Build history of the part. All positions in model axes, mm. A direction names the side the tool comes from. Give positions to 0.01 mm unless a question says otherwise; leave off trailing zeros. Order: outer loops, then holes, each group sorted by start corner. A loop starts at its lowest first (then second) coordinate and runs counter-clockwise, first axis right, second up. Notation, with made-up numbers: (51.5, -0.75) -> (95.5, -0.75) arc R10 ccw to (95.5, 16.25) -> close; hole circle Ø1 at (-30.75, -28). An arc over 180 degrees is marked (long way). One line per item, written item: value. Start each with the question number.
(1) Which spindle directions (+Z, -Z, +X, -X, +Y, -Y) get a long thin tool onto all of the face, cutting with end or side? Do faces 1 (the flat face through (272.5, 276, 290)), 2 (the flat face through (272.5, 324, 290)), 3 (the cylindrical face through (269.78, 284.43, 289.96)), 4 (the flat face through (267, 326, 307)), 5 (the flat face through (269.5, 300, 310)). Say none if no direction does.
(2) Two-plate mould, pull along Z, no slides. Class faces 6 (the flat face through (272.5, 300, 290)), 7 (the flat face through (268, 300, 287)), 8 (the flat face through (270, 300, 293)): +Z half, -Z half, draft (parallel to the pull), parting line (faces both ways), or undercut.
(3) Probe line 1 (Y direction, x = 267.25, z = 300); line 2 (Z direction, x = 265.85, y = 300); line 3 (Y direction, x = 265.2, z = 293.25). List the from-to ranges inside material, lowest first.
(4) Saw through at C-C on y = 300. Give the cut face in (x, z).
(5) Saw through at A-A on y = 283. Give the cut face in (x, z).
(6) Pin check, flat tips, straight feed: pin 1 (4 mm diameter, centred on y = 311.69, z = 293.25, fed in from +X); pin 2 (3 mm diameter, centred on y = 303.5, z = 309, fed in from +X); pin 3 (3.5 mm diameter, centred on y = 276, z = 289, fed in from +X); pin 4 (2 mm diameter, centred on x = 270.7, y = 317, fed in from +Z). Stop position of each tip, or through.
(7) Saw through at B-B on z = 313.5. Give the cut face in (x, y).
(8) Saw through at D-D on x = 267.5. Give the cut face in (y, z).
```python
from build123d import *

# Parameters (mm, degrees)
SKETCH1_W           = 39.5
SKETCH1_H           = 52
SKETCH1_R           = 1.45
BOSS_EXTRUDE1_DEPTH = 5.5
SKETCH2_R           = 7.6
CUT_EXTRUDE1_DEPTH  = 5.5
SKETCH3_W           = 8.5
SKETCH3_H           = 52
BOSS_EXTRUDE2_DEPTH = 6
SKETCH4_R           = 5.05
SKETCH4_R_2         = 1.7
BOSS_EXTRUDE3_DEPTH = 6
SKETCH5_R           = 5.05
SKETCH5_R_2         = 1.7
BOSS_EXTRUDE4_DEPTH = 6
SKETCH6_R           = 1.7
CUT_EXTRUDE2_DEPTH  = 6


with BuildPart() as part:
    # Sketch1 → Boss-Extrude1 (new body)
    with BuildSketch(Plane(origin=(264, 0, 0), x_dir=(0, 0, -1), z_dir=(1, 0, 0))):
        with Locations((-306.75, 300)):
            Rectangle(SKETCH1_W, SKETCH1_H)
        with Locations((-313.5, 300)):
            Circle(SKETCH1_R, mode=Mode.SUBTRACT)
        with Locations((-293.25, 311.691342951)):
            Circle(SKETCH1_R, mode=Mode.SUBTRACT)
        with Locations((-293.25, 288.308657049)):
            Circle(SKETCH1_R, mode=Mode.SUBTRACT)
    extrude(amount=BOSS_EXTRUDE1_DEPTH)

    # Sketch2 → Cut-Extrude1 (cut)
    with BuildSketch(Plane(origin=(264, 0, 0), x_dir=(0, 0, -1), z_dir=(1, 0, 0))):
        with Locations((-300, 300)):
            Circle(SKETCH2_R)
    extrude(amount=CUT_EXTRUDE1_DEPTH, mode=Mode.SUBTRACT)

    # Sketch3 → Boss-Extrude2 (add)
    with BuildSketch(Plane.XY.offset(287)):
        with Locations((268.25, 300)):
            Rectangle(SKETCH3_W, SKETCH3_H)
    extrude(amount=BOSS_EXTRUDE2_DEPTH)

    # Sketch4 → Boss-Extrude3 (add)
    with BuildSketch(Plane.XY.offset(287)):
        with Locations((270.7, 283)):
            Circle(SKETCH4_R)
        with Locations((270.7, 283)):
            Circle(SKETCH4_R_2, mode=Mode.SUBTRACT)
    extrude(amount=BOSS_EXTRUDE3_DEPTH)

    # Sketch5 → Boss-Extrude4 (add)
    with BuildSketch(Plane.XY.offset(287)):
        with Locations((270.7, 317)):
            Circle(SKETCH5_R)
        with Locations((270.7, 317)):
            Circle(SKETCH5_R_2, mode=Mode.SUBTRACT)
    extrude(amount=BOSS_EXTRUDE4_DEPTH)

    # Sketch6 → Cut-Extrude2 (cut)
    with BuildSketch(Plane.XY.offset(287)):
        with Locations(Location((270.7, 283, 0), (0, 0, 225.099127844))):
            Circle(SKETCH6_R)
        with Locations(Location((270.7, 317, 0), (0, 0, 225.099127844))):
            Circle(SKETCH6_R)
    extrude(amount=CUT_EXTRUDE2_DEPTH, mode=Mode.SUBTRACT)


solid = part.part
```
Results below:
1. face 1: +Z, -Z, +X, -Y
1. face 2: +Z, -Z, +X, +Y
1. face 3: -Z
1. face 4: +Z, -Z, +X, -X, +Y
1. face 5: +Z, +X, +Y, -Y
2. face 6: draft
2. face 7: -Z half
2. face 8: undercut
3. line 1: y = 274 to 292.4, 307.6 to 326
3. line 2: z = 287 to 293, 307.6 to 312.05, 314.95 to 326.5
3. line 3: y = 274 to 286.86, 289.76 to 296.51, 303.49 to 310.24, 313.14 to 326
4. outline: (264, 287) -> (272.5, 287) -> (272.5, 293) -> (264, 293) -> close; (264, 307.6) -> (269.5, 307.6) -> (269.5, 312.05) -> (264, 312.05) -> close; (264, 314.95) -> (269.5, 314.95) -> (269.5, 326.5) -> (264, 326.5) -> close
5. outline: (264, 287) -> (269, 287) -> (269, 293) -> (269.5, 293) -> (269.5, 326.5) -> (264, 326.5) -> close; (272.4, 287) -> (275.75, 287) -> (275.75, 293) -> (272.4, 293) -> close
6. pin 1: stops at x = 274.5
6. pin 2: stops at x = 269.5
6. pin 3: stops at x = 272.5
6. pin 4: passes through
7. outline: (264, 274) -> (269.5, 274) -> (269.5, 298.55) -> (264, 298.55) -> close; (264, 301.45) -> (269.5, 301.45) -> (269.5, 326) -> (264, 326) -> close
8. outline: (274, 287) -> (326, 287) -> (326, 326.5) -> (274, 326.5) -> close; hole (286.88, 293) -> (289.74, 293) arc R1.45 ccw (long way) to start; hole (297.04, 293) -> (302.96, 293) arc R7.6 ccw (long way) to start; hole circle Ø2.9 at (300, 313.5); hole (310.26, 293) -> (313.12, 293) arc R1.45 ccw (long way) to start
